Source: CAD feature listing. Evaluate the final solid. Frame: model axes, mm. Face numbers are marked on the shaded views. A direction names the side the tool comes from. Round coordinates to 2 decimals unless told otherwise and drop trailing zeros. Loops run counter-clockwise (first coordinate to the right, second up) from the corner with the lowest first, then second, coordinate; pieces in that order, holes last.
Item 1: Access query for the marked faces 1 and 2. Directions: +Z, -Z, +X, -X, +Y, -Y. A direction counts if a zero-diameter tool reaches every point of the face in a straight line with its end or side. Return the directions, or none.
Item 2: Section query C-C on x = -32.5. Return loops of the section in (y, z).
Item 3: Pull-direction query (X, two-part tool) for the marked faces 3 and 4; classes: released by +X, released by -X, zero draft, split by the parting line, or undercut.
Item 4: Section query A-A on z = 5. Return loops of the section in (x, y).
Item 5: Section query B-B on x = 13. Return loops of the section in (y, z), then the cut area to 3 significant figures.
Item 6: Ray query, L1, parallel to X at y = -35.8, z = 5; L2, parallel to Y at x = -72, z = 6.25; L3, parallel to X at y = -34.55, z = 5. Return the intervals inside material, ascending.
Item 7: First-contact query: P1, Ø6, axis at x = -5.5, y = 7.5, coming from the -Z side; P2, Ø4, axis at y = -28.5, z = 8, coming from the -X side; P3, Ø5, axis at x = 28, z = 5.5, coming from the +Y side; P4, Ø3, axis at y = 0.5, z = 2, coming from the +X side. Flat tips, straight axial feed; report the tip coordinate or a pass-through.
```python
from build123d import *

# Parameters (mm, degrees)
SKETCH1_R           = 2.25
SKETCH1_W           = 21
SKETCH1_H           = 41
BOSS_EXTRUDE1_DEPTH = 10
SKETCH1_3_R         = 2.25
CUT_EXTRUDE1_DEPTH  = 10
SKETCH2_R           = 1.5
CUT_EXTRUDE2_DEPTH  = 5
FILLET1_R           = 2
FILLET2_R           = 2


with BuildPart() as part:
    # Sketch1 → Boss-Extrude1 (new body)
    # profile 1 of 3: a face of its own
    with BuildSketch(Plane.XY):
        Polygon((38.094892468, -32.802015288), (8.094892468, -32.802015288), (-16.905107532, 23.197984712), (-36.905107532, 23.197984712), (-61.905107532, -32.802015288), (-91.905107532, -32.802015288), (-91.905107532, -37.802015288), (38.094892468, -37.802015288), align=None)
        with Locations((-20.905107532, -32.802015288)):
            Circle(SKETCH1_R, mode=Mode.SUBTRACT)
        with Locations((-31.905107532, 18.197984712)):
            Circle(SKETCH1_R, mode=Mode.SUBTRACT)
        with Locations((-26.405107532, -7.302015288)):
            Rectangle(SKETCH1_W, SKETCH1_H, mode=Mode.SUBTRACT)
    # profile 2 of 3: a face of its own
    with BuildSketch(Plane.XY):
        with Locations((-31.905107532, 18.197984712)):
            Circle(SKETCH1_R)
    # profile 3 of 3: a face of its own
    with BuildSketch(Plane.XY):
        with Locations((-20.905107532, -32.802015288)):
            Circle(SKETCH1_R)
    extrude(amount=BOSS_EXTRUDE1_DEPTH)

    # Sketch1_3 → Cut-Extrude1 (cut)
    with BuildSketch(Plane.XY):
        with Locations((-31.905107532, 18.197984712)):
            Circle(SKETCH1_3_R)
        with Locations((-20.905107532, -32.802015288)):
            Circle(SKETCH1_3_R)
    extrude(amount=CUT_EXTRUDE1_DEPTH, mode=Mode.SUBTRACT)

    # Sketch2 → Cut-Extrude2 (cut)
    with BuildSketch(Plane(origin=(0, -32.802015288, 0), x_dir=(1, 0, 0), z_dir=(0, 1, 0))):
        with Locations(Location((33.094892468, -5, 0), (0, 0, 270))):
            Circle(SKETCH2_R)
        with Locations(Location((-86.905107532, -5, 0), (0, 0, 270))):
            Circle(SKETCH2_R)
    extrude(amount=-CUT_EXTRUDE2_DEPTH, mode=Mode.SUBTRACT)

    # Fillet1
    fillet1_edges = [part.edges().sort_by_distance(p)[0] for p in [
        (-61.905107532, -32.802015288, 5),
        (-36.905107532, 23.197984712, 5),
        (-16.905107532, 23.197984712, 5),
        (8.094892468, -32.802015288, 5),
    ]]
    fillet(fillet1_edges, radius=FILLET1_R)

    # Fillet2
    fillet2_edges = [part.edges().sort_by_distance(p)[0] for p in [
        (-26.905107532, -37.802015288, 0),
        (23.743588762, -32.802015288, 0),
        (23.743588762, -32.802015288, 10),
        (-26.905107532, -37.802015288, 10),
        (-77.553803825, -32.802015288, 0),
        (-77.553803825, -32.802015288, 10),
        (-49.405107532, -4.802015288, 0),
        (-49.405107532, -4.802015288, 10),
        (-4.405107532, -4.802015288, 0),
        (-4.405107532, -4.802015288, 10),
        (-26.905107532, 23.197984712, 0),
        (-17.114061641, 22.875870787, 0),
        (-36.696153423, 22.875870787, 0),
        (-26.905107532, 23.197984712, 10),
        (-17.114061641, 22.875870787, 10),
        (-36.696153423, 22.875870787, 10),
        (-62.114061641, -32.479901363, 0),
        (-62.114061641, -32.479901363, 10),
        (8.303846577, -32.479901363, 0),
        (8.303846577, -32.479901363, 10),
    ]]
    fillet(fillet2_edges, radius=FILLET2_R)


solid = part.part
```
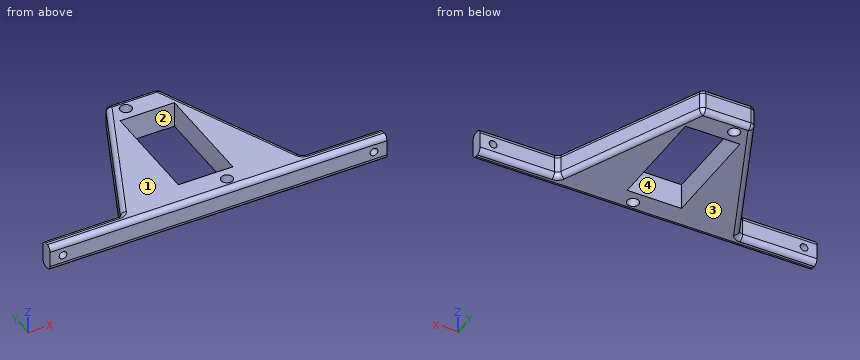
Data:
1. face 1: +Z, +X, -X, +Y, -Y
1. face 2: +Z, -Z
2. outline: (-37.8, 2) arc R2 ccw to (-35.8, 0) - (-27.8, 0) - (-27.8, 10) - (-35.8, 10) arc R2 ccw to (-37.8, 8) - close; (13.2, 0) - (16.03, 0) - (16.03, 10) - (13.2, 10) - close; (20.37, 0) - (21.2, 0) arc R2 ccw to (23.2, 2) - (23.2, 8) arc R2 ccw to (21.2, 10) - (20.37, 10) - close
3. face 3: zero draft
3. face 4: undercut
4. outline: (-91.91, -37.8) - (-88.41, -37.8) - (-88.41, -32.8) - (-91.91, -32.8) - close; (-85.41, -37.8) - (31.59, -37.8) - (31.59, -32.8) - (9.39, -32.8) arc R2 cw to (7.57, -31.62) - (-16.38, 22.01) arc R2 ccw to (-18.2, 23.2) - (-35.61, 23.2) arc R2 ccw to (-37.43, 22.01) - (-61.38, -31.62) arc R2 cw to (-63.2, -32.8) - (-85.41, -32.8) - close; (34.59, -37.8) - (38.09, -37.8) - (38.09, -32.8) - (34.59, -32.8) - close; hole (-36.91, -27.8) - (-15.91, -27.8) - (-15.91, 13.2) - (-36.91, 13.2) - close; hole circle Ø4.5 at (-31.91, 18.2); hole circle Ø4.5 at (-20.91, -32.8)
5. outline: (-37.8, 2) arc R2 ccw to (-35.8, 0) - (-34.8, 0) arc R2 ccw to (-32.8, 2) - (-32.8, 8) arc R2 ccw to (-34.8, 10) - (-35.8, 10) arc R2 ccw to (-37.8, 8) - close
5. area: 46.6 mm2
6. L1: x = -91.91 to -88.41, -85.41 to 31.59, 34.59 to 38.09
6. L2: y = -37.8 to -32.8
6. L3: x = -91.91 to -88.41, -85.41 to -22.32, -19.49 to 31.59, 34.59 to 38.09
7. P1: passes through
7. P2: stops at x = -60.88
7. P3: stops at y = -32.8
7. P4: stops at x = -6.1
